Source: CAD feature listing. Evaluate the final solid. Frame: model axes, mm. A direction names the side the tool comes from. Round coordinates to 2 decimals unless told otherwise and drop trailing zeros. Order: outer loops, then holes, each group sorted by start corner. A loop starts at its lowest first (then second) coordinate and runs counter-clockwise, first axis right, second up. Notation, with made-up numbers: M 55,7 L 87,7 A28 ccw 87,35 Z; hole C 19.5,89.5 d4. An arc over 180 degrees is marked long. Use one line per item in the form item = value. Start each with the question number.
Q1. Section C-C (x = 3.5). Return the cut outline in (y, z), plus the area to 3 significant figures.
Q2. Section B-B (z = -0.5). Return the cut outline in (x, y).
Q3. Material intervals for probe 1 along Z at (x, y) = (-1.75, -1.25); probe 2 along X at (y, z) = (-0.2, 1.5); probe 3 along X at (y, z) = (0.1, -4), sorted ascending.
Q4. Pull-direction query (X, two-part tool) for faces 3 (the flat face through (8, 0, 0)), 4 (the cylindrical face through (-3.93, 0.02, 3.9)), 5 (the flat face through (0, 1.5, -5)); classes: pulls with the +X half, pulls with the -X half, needs draft (parallel to the pull), parting line crosses it, or undercut.
Q5. Reachability of faces 1 (the flat face through (0, 0, 4.5)), 2 (the flat face through (0, 0, 11)) from +Z, -Z, +X, -X, +Y, -Y: full face, straight path, thin tool, end or side. Return the list, or none.
Q6. Section A-A (y = 1.15). Return the cut outline in (x, z).
from build123d import *

# Parameters (mm, degrees)
SKETCH1_W           = 16
SKETCH1_H           = 22
SKETCH1_W_2         = 9
SKETCH1_H_2         = 9
BOSS_EXTRUDE1_DEPTH = 1.5
FILLET1_R           = 2


with BuildPart() as part:
    # Sketch1 → Boss-Extrude1 (new body, symmetric)
    with BuildSketch(Plane(origin=(0, 0, 0), x_dir=(1, 0, 0), z_dir=(0, 1, 0))):
        Rectangle(SKETCH1_W, SKETCH1_H)
        Rectangle(SKETCH1_W_2, SKETCH1_H_2, mode=Mode.SUBTRACT)
    extrude(amount=BOSS_EXTRUDE1_DEPTH, both=True)

    # Fillet1
    fillet1_edges = [part.edges().sort_by_distance(p)[0] for p in [
        (-4.5, 0, -4.5),
        (-4.5, 0, 4.5),
        (4.5, 0, 4.5),
        (4.5, 0, -4.5),
    ]]
    fillet(fillet1_edges, radius=FILLET1_R)


solid = part.part
Results list:
q1.outline = M -1.5,-11 L 1.5,-11 L 1.5,-4.23 L -1.5,-4.23 Z; M -1.5,4.23 L 1.5,4.23 L 1.5,11 L -1.5,11 Z
q1.area = 40.6 mm2
q2.outline = M -8,-1.5 L -4.5,-1.5 L -4.5,1.5 L -8,1.5 Z; M 4.5,-1.5 L 8,-1.5 L 8,1.5 L 4.5,1.5 Z
q3.probe_1 = -11 to -4.5, 4.5 to 11
q3.probe_2 = -8 to -4.5, 4.5 to 8
q3.probe_3 = -8 to -3.82, 3.82 to 8
q4.face_3 = pulls with the +X half
q4.face_4 = undercut
q4.face_5 = needs draft
q5.face_1 = +Y, -Y
q5.face_2 = +Z, +X, -X, +Y, -Y
q6.outline = M -8,-11 L 8,-11 L 8,11 L -8,11 Z; hole M -4.5,-2.5 A2 ccw -2.5,-4.5 L 2.5,-4.5 A2 ccw 4.5,-2.5 L 4.5,2.5 A2 ccw 2.5,4.5 L -2.5,4.5 A2 ccw -4.5,2.5 Z
